Verification items for the finished model (mm, model axes). A direction names the side the tool comes from. Give positions to 0.01 mm unless a question says otherwise; leave off trailing zeros. Write each loop counter-clockwise with the first axis right and the second up, starting at its lowest first coordinate (ties: lowest second). Pieces come first, ordered by that corner, then holes. Notation, with made-up numbers: (-8, 66) -> (14, 66) arc R10 cw to (14, 77) -> close; hole circle Ø9 at (-15.75, -0.5). An arc over 180 degrees is marked (long way). Use one line per item in the form item = value. Start each with the question number.
(1) Depth check by flat-ended pin: pin 1 Ø1.3 at (x, z) = (-12, -67.5) entering from -Y; pin 2 Ø2.5 at (x, y) = (-1, -1) entering from -Z; pin 3 Ø0.9 at (x, y) = (0, 4.5) entering from -Z; pin 4 Ø1.3 at (y, z) = (-2.5, -68.5) entering from -X. Enter the tip coordinate at first touch or a pass-through.
(2) Scan lines: L1, parallel to Z at x = 28, y = -1.25; L2, parallel to X at y = -2, z = 62; L3, parallel to Z at x = 0, y = 2.1. Record each from-to range of solid material in increasing order.
(3) Section check B-B, the plane x = 0. State how many separate pieces and enclosed holes the cut face has, plus the area to 3 significant figures.
(4) Section check A-A, the plane z = 60. Record the cut outline in (x, y).
(5) Section check C-C, the plane x = -17.5. Record the cut outline in (y, z).
(6) Set-up check for faces 4 (the face through (27.254, 2, 59)), 5 (the face through (32.194, -0.036, -65.801)), 6 (the face through (-24.959, -2, -68)): record each of +Z, -Z, +X, -X, +Y, -Y from which the full face is reachable in a straight line by a thin tool's end or side.
(7) Section check D-D, the plane z = 17.5. Record the cut outline in (x, y), plus the area to 3 significant figures.
(8) Release check for a two-part mould opening along X. For faces 1 (the face through (0, 4, -17.264)), 2 (the face through (0, 0, 69.15)), 3 (the face through (-32.12, -0.05, -67.65)) record: pulls with the +X half, pulls with the -X half, needs draft (parallel to the pull), parting line crosses it, or undercut.
from build123d import *

# Parameters (mm, degrees)
F0_W          = 67.1
F0_H          = 138.3
F1_DEPTH      = 3.55
F2_T          = -2.54
F3_R          = 5
F4_W          = 16.3524625823
F4_H          = 7.4590183794
F5_DEPTH      = 12.5
F6_W          = 49.3442639709
F6_H          = 3.55
F7_DEPTH      = 12.5
F8_R          = 11.5647163982
F9_DEPTH      = 12.5
F10_W         = 6
F10_H         = 10
F11_DEPTH     = 2
F12_T         = 1
F12_T3_DEPTH  = 12
F12_T5_DEPTH  = 8
F12_T7_DEPTH  = 4.54
F12_T9_DEPTH  = 4.54
F12_T11_DEPTH = 6.56
F12_T13_DEPTH = 64.02
F12_T15_DEPTH = 135.22


# Not quite as in the source:
# - a shell that OpenCascade refuses in one call is made with other operations: the cavity is built on its own and cut out


with BuildPart() as f1:
    # F0 (on Front) → F1 (new body, symmetric)
    with BuildSketch(Plane.XZ):
        Rectangle(F0_W, F0_H)
    extrude(amount=F1_DEPTH, both=True)

    # F2
    f2_openings = [f1.faces().sort_by_distance(p)[0] for p in [
        (0, -3.55, 0),
    ]]
    offset(amount=F2_T, openings=f2_openings)

    # F3
    f3_edges = [f1.edges().sort_by_distance(p)[0] for p in [
        (-33.55, 0, 69.15),
        (-33.55, 0, -69.15),
        (33.55, 0, 69.15),
        (33.55, 0, -69.15),
    ]]
    fillet(f3_edges, radius=F3_R)

    # F4 (on face) → F5 (cut, symmetric)
    with BuildSketch(Plane.XZ.offset(-1.01)):
        with Locations((19.0778714605, 59.2418070883)):
            Rectangle(F4_W, F4_H)
    extrude(amount=F5_DEPTH, both=True, mode=Mode.SUBTRACT)

    # F6 (on face) → F7 (cut, symmetric)
    with BuildSketch(Plane(origin=(0, 0, -69.15), x_dir=(1, 0, 0), z_dir=(0, 0, -1))):
        with Locations((-0.2868864685, 1.775)):
            Rectangle(F6_W, F6_H)
    extrude(amount=F7_DEPTH, both=True, mode=Mode.SUBTRACT)

    # F8 (on face) → F9 (cut, symmetric)
    with BuildSketch(Plane.XZ.offset(-1.01)):
        with Locations((0, 31.700823456)):
            Circle(F8_R)
    extrude(amount=F9_DEPTH, both=True, mode=Mode.SUBTRACT)

    # F10 (on face) → F11 (join)
    with BuildSketch(Plane(origin=(0, 3.55, 0), x_dir=(-1, 0, 0), z_dir=(0, 1, 0))):
        with Locations((0.4249104531, -21.26386761)):
            Rectangle(F10_W, F10_H)
    extrude(amount=F11_DEPTH)

    # F12: shell of thickness 1, made by hand


with BuildPart() as f12_core1:
    # F12_t2: copy of F1
    add(f1.part)

    # the walls: a layer under each face that stays
    f12_faces = [f12_core1.faces().sort_by_distance(p)[0] for p in [
        (0, 0, 69.15),
        (0, 3.55, 0),
        (32.0855339059, 0, 67.6855339059),
        (-32.0855339059, 0, 67.6855339059),
        (-31.3133333333, -3.55, -64.54),
        (33.55, 0, 0),
        (-33.55, 0, 0),
        (32.0855339059, 0, -67.6855339059),
        (-32.0855339059, 0, -67.6855339059),
        (-19.0333333333, 2.3666666667, -69.15),
        (-3.4249104531, 4.55, -21.26386761),
        (-0.4249104531, 4.55, -26.26386761),
        (2.5750895469, 4.55, -21.26386761),
        (-0.4249104531, 4.55, -16.26386761),
        (-11.5647163982, 2.28, 31.700823456),
        (19.0778714605, 2.28, 62.971316278),
        (27.2541027516, 2.28, 59.2418070883),
        (10.9016401693, 2.28, 59.2418070883),
        (19.0778714605, 2.28, 55.5122978985),
        (24.3852455169, -1.775, -67.88),
        (-20.6733333333, 0.25, -66.61),
        (31.01, -1.27, 0),
        (0, -1.27, 66.61),
        (-31.01, -1.27, 0),
        (-24.959018454, -1.775, -67.88),
        (-0.2868864685, 0, -67.88),
        (0, 1.01, 0),
    ]]
    thicken(f12_faces, amount=-F12_T, mode=Mode.SUBTRACT)

    # F12_s4 → F12_t3 (cut)
    with BuildSketch(Plane.XY.offset(-27.26386761)):
        Polygon((-3.4349104531, 3.56), (-3.4249104531, 2.55), (-2.4249104531, 2.55), (-2.4249104531, 3.55), align=None)
        Polygon((2.5850895469, 3.56), (2.5750895469, 2.55), (1.5750895469, 2.55), (1.5750895469, 3.55), align=None)
    extrude(amount=F12_T3_DEPTH, mode=Mode.SUBTRACT)

    # F12_s6 → F12_t5 (cut)
    with BuildSketch(Plane.YZ.offset(-4.4249104531)):
        Polygon((3.56, -26.27386761), (2.55, -26.26386761), (2.55, -25.26386761), (3.55, -25.26386761), align=None)
        Polygon((3.56, -16.25386761), (2.55, -16.26386761), (2.55, -17.26386761), (3.55, -17.26386761), align=None)
    extrude(amount=F12_T5_DEPTH, mode=Mode.SUBTRACT)

    # F12_s8 → F12_t7 (cut)
    with BuildSketch(Plane.XZ.offset(-4.55)):
        Polygon((27.2441027516, 62.961316278), (27.2541027516, 63.971316278), (28.2541027516, 63.971316278), (28.2541027516, 62.971316278), align=None)
        Polygon((10.9116401693, 62.961316278), (10.9016401693, 63.971316278), (9.9016401693, 63.971316278), (9.9016401693, 62.971316278), align=None)
        Polygon((27.2441027516, 55.5222978985), (28.2541027516, 55.5122978985), (28.2541027516, 54.5122978985), (27.2541027516, 54.5122978985), align=None)
        Polygon((10.9116401693, 55.5222978985), (9.9016401693, 55.5122978985), (9.9016401693, 54.5122978985), (10.9016401693, 54.5122978985), align=None)
    extrude(amount=F12_T7_DEPTH, mode=Mode.SUBTRACT)

    # F12_s10 → F12_t9 (cut)
    with BuildSketch(Plane.XY.offset(-70.15)):
        Polygon((24.3752455169, -0.01), (25.3852455169, 0), (25.3852455169, 1), (24.3852455169, 1), align=None)
        Polygon((-24.949018454, -0.01), (-25.959018454, 0), (-25.959018454, 1), (-24.959018454, 1), align=None)
    extrude(amount=F12_T9_DEPTH, mode=Mode.SUBTRACT)

    # F12_s12 → F12_t11 (cut)
    with BuildSketch(Plane.XZ.offset(-2.01)):
        Polygon((31, -66.6), (31.01, -67.61), (32.01, -67.61), (32.01, -66.61), align=None)
        Polygon((-31, -66.6), (-31.01, -67.61), (-32.01, -67.61), (-32.01, -66.61), align=None)
        Polygon((31, 66.6), (32.01, 66.61), (32.01, 67.61), (31.01, 67.61), align=None)
        Polygon((-31, 66.6), (-31.01, 67.61), (-32.01, 67.61), (-32.01, 66.61), align=None)
    extrude(amount=F12_T11_DEPTH, mode=Mode.SUBTRACT)

    # F12_s14 → F12_t13 (cut)
    with BuildSketch(Plane.YZ.offset(-32.01)):
        Polygon((1, -66.6), (1.01, -67.61), (2.01, -67.61), (2.01, -66.61), align=None)
        Polygon((1, 66.6), (1.01, 67.61), (2.01, 67.61), (2.01, 66.61), align=None)
    extrude(amount=F12_T13_DEPTH, mode=Mode.SUBTRACT)

    # F12_s16 → F12_t15 (cut)
    with BuildSketch(Plane.XY.offset(-67.61)):
        Polygon((31, 1), (32.01, 1.01), (32.01, 2.01), (31.01, 2.01), align=None)
        Polygon((-31, 1), (-32.01, 1.01), (-32.01, 2.01), (-31.01, 2.01), align=None)
    extrude(amount=F12_T15_DEPTH, mode=Mode.SUBTRACT)


with BuildPart() as f1_1:
    add(f1.part)

    # what is left inside the walls is the cavity
    f12_cavity = [f12_core1.part.solids().sort_by_distance(p)[0] for p in [
        (-16.275, 2.54, 22.716667),
    ]]
    add(f12_cavity, mode=Mode.SUBTRACT)


solid = f1_1.part
Completed:
q1.pin_1 = 0
q1.pin_2 = -69.15
q1.pin_3 = -26.26
q1.pin_4 = -31.91
q2.L1 = -69.15 to -68.15, -67.61 to -66.61, 66.61 to 67.61, 68.15 to 69.15
q2.L2 = -33.55 to -32.55, -32.01 to -31.01, 31.01 to 32.01, 32.55 to 33.55
q2.L3 = -69.15 to -68.15, 19.14 to 20.14, 43.27 to 44.27, 68.15 to 69.15
q3.separate_pieces = 2
q3.enclosed_holes = 1
q3.area = 240 mm²
q4.outline = (-33.55, -3.55) -> (-31.01, -3.55) -> (-31.01, 1.01) -> (10.9, 1.01) -> (10.9, 3.55) -> (-33.55, 3.55) -> close; (27.25, 1.01) -> (31.01, 1.01) -> (31.01, -3.55) -> (33.55, -3.55) -> (33.55, 3.55) -> (27.25, 3.55) -> close; hole (-32.55, -2.55) -> (-32.01, -2.55) -> (-32.01, 2.01) -> (9.9, 2.01) -> (9.9, 2.55) -> (-32.55, 2.55) -> close; hole (28.25, 2.01) -> (32.01, 2.01) -> (32.01, -2.55) -> (32.55, -2.55) -> (32.55, 2.55) -> (28.25, 2.55) -> close
q5.outline = (-3.55, 66.61) -> (1.01, 66.61) -> (1.01, -66.61) -> (0, -66.61) -> (0, -69.15) -> (3.55, -69.15) -> (3.55, 69.15) -> (-3.55, 69.15) -> close; hole (-2.55, 67.61) -> (2.01, 67.61) -> (2.01, -67.61) -> (1, -67.61) -> (1, -68.15) -> (2.55, -68.15) -> (2.55, 68.15) -> (-2.55, 68.15) -> close
q6.face_4 = +Y, -Y
q6.face_5 = none
q6.face_6 = -Z, -Y
q7.outline = (-33.55, -3.55) -> (-31.01, -3.55) -> (-31.01, 1.01) -> (31.01, 1.01) -> (31.01, -3.55) -> (33.55, -3.55) -> (33.55, 3.55) -> (-33.55, 3.55) -> close; hole (-32.55, -2.55) -> (-32.01, -2.55) -> (-32.01, 2.01) -> (32.01, 2.01) -> (32.01, -2.55) -> (32.55, -2.55) -> (32.55, 2.55) -> (-32.55, 2.55) -> close
q7.area = 154 mm²
q8.face_1 = undercut
q8.face_2 = needs draft
q8.face_3 = pulls with the -X half
